```python
from build123d import *

# Parameters (mm, degrees)
F0_R     = 2.75
F0_R_2   = 1.625
F1_DEPTH = 6


with BuildPart() as f1:
    # F0 (on Top) → F1 (new body)
    with BuildSketch(Plane.XY):
        Polygon((-6, 15), (-15.5, 15), (-15.5, 26), (-25.5, 26), (-25.5, 15), (-25.5, 0), (-22.25, -52), (-9.25, -52), (-9.25, -45.5), (-11.5, -6.5), (-11.5, 0), (11.5, 0), (11.5, -6.5), (9.25, -45.5), (9.25, -52), (22.25, -52), (25.5, 0), (25.5, 15), (25.5, 26), (15.5, 26), (15.5, 15), (6, 15), (6, 8), (-6, 8), align=None)
        with Locations((-15.75, -45.5)):
            Circle(F0_R, mode=Mode.SUBTRACT)
        with Locations((-15, -33)):
            Circle(F0_R_2, mode=Mode.SUBTRACT)
        with Locations((15.75, -45.5)):
            Circle(F0_R, mode=Mode.SUBTRACT)
        with Locations((15, -33)):
            Circle(F0_R_2, mode=Mode.SUBTRACT)
        with Locations((-15, -3)):
            Circle(F0_R_2, mode=Mode.SUBTRACT)
        with Locations((-17, 6.5)):
            Circle(F0_R, mode=Mode.SUBTRACT)
        with Locations((15, -3)):
            Circle(F0_R_2, mode=Mode.SUBTRACT)
        with Locations((17, 6.5)):
            Circle(F0_R, mode=Mode.SUBTRACT)
    extrude(amount=F1_DEPTH)


solid = f1.part
```
Geometry check sheet. Reference: the model listing, model coordinates, mm. A direction names the side the tool comes from. Give positions to 0.01 mm unless a question says otherwise; leave off trailing zeros. Loops run counter-clockwise (first coordinate to the right, second up) from the corner with the lowest first, then second, coordinate; pieces in that order, holes last. Notation, with made-up numbers: M 77,-13 L 100,-13 A20 cw 100,-3 Z; hole C 35.25,36.25 d10. An arc over 180 degrees is marked long. Write item = value, one per line.
(1) Release check for a two-part mould opening along X. For faces 1 (the face through (-23.9, -25.6, 3)), 2 (the face through (-20, 26, 3)), 3 (the face through (-9.25, -49, 3)) record: released by +X, released by -X, zero draft, split by the parting line, or undercut.
Answer below:
face_1 = released by -X
face_2 = zero draft
face_3 = undercut
(2) Sectioned sample at A-A, the plane y = 6.5. Record the cut outline in (x, z).
Answer below:
outline = M -25.5,0 L -19.75,0 L -19.75,6 L -25.5,6 Z; M -14.25,0 L 14.25,0 L 14.25,6 L -14.25,6 Z; M 19.75,0 L 25.5,0 L 25.5,6 L 19.75,6 Z
(3) Gauge pin test, flat ends, axial feed: pin 1 Ø1.9 at (x, y) = (15, -3) entering from -Z; pin 2 Ø3 at (x, z) = (-10, 1.5) entering from +Y; pin 3 Ø6.5 at (x, y) = (-17, 6.5) entering from +Z; pin 4 Ø1.8 at (x, z) = (4.5, 4.5) entering from -Y. Record the tip position at first contact, or that the pin passes through.
Answer below:
pin_1 = through
pin_2 = 15
pin_3 = 6
pin_4 = 0
(4) Sectioned sample at D-D, the plane y = -33. Record the cut outline in (x, z) (1 decimal).
Answer below:
outline = M -23.4,0 L -16.6,0 L -16.6,6 L -23.4,6 Z; M -13.4,0 L -10,0 L -10,6 L -13.4,6 Z; M 10,0 L 13.4,0 L 13.4,6 L 10,6 Z; M 16.6,0 L 23.4,0 L 23.4,6 L 16.6,6 Z
(5) Sectioned sample at C-C, the plane y = 21. Record the cut outline in (x, z), plus the area to 3 significant figures.
Answer below:
outline = M -25.5,0 L -15.5,0 L -15.5,6 L -25.5,6 Z; M 15.5,0 L 25.5,0 L 25.5,6 L 15.5,6 Z
area = 120 mm2
(6) Sectioned sample at B-B, the plane z = 2.25. State how many separate pieces and enclosed holes the cut face has, plus the area to 3 significant figures.
Answer below:
separate_pieces = 1
enclosed_holes = 8
area = 2,180 mm2
(7) Tool access check on faces 4 (the face through (-12, -12, 6)), 5 (the face through (0, 0, 3)), 6 (the face through (0, 8, 3)), 7 (the face through (9.25, -49, 3)), 8 (the face through (16, -52, 3)). Record the directions out of +Z, -Z, +X, -X, +Y, -Y that give a thin tool (end or side, any length) a straight path to the whole face; none if there is none.
Answer below:
face_4 = +Z, +X, -X, +Y, -Y
face_5 = +Z, -Z
face_6 = +Z, -Z, +Y
face_7 = +Z, -Z, -Y
face_8 = +Z, -Z, +X, -X, -Y
(8) Material ranges on line 1 (X direction, y = 9, z = 4.35); line 2 (Y direction, x = -15, z = 3.25) (3 decimals); line 3 (Y direction, x = -15.75, z = 1.8), recorded low to high. Write a range as [from, to].
Answer below:
line_1 = [-25.5, -18.15], [-15.85, -6], [6, 15.85], [18.15, 25.5]
line_2 = [-52, -48.146], [-42.854, -34.625], [-31.375, -4.625], [-1.375, 4.613], [8.387, 15]
line_3 = [-52, -48.25], [-42.75, -34.44], [-31.56, -4.44], [-1.56, 4.05], [8.95, 26]
